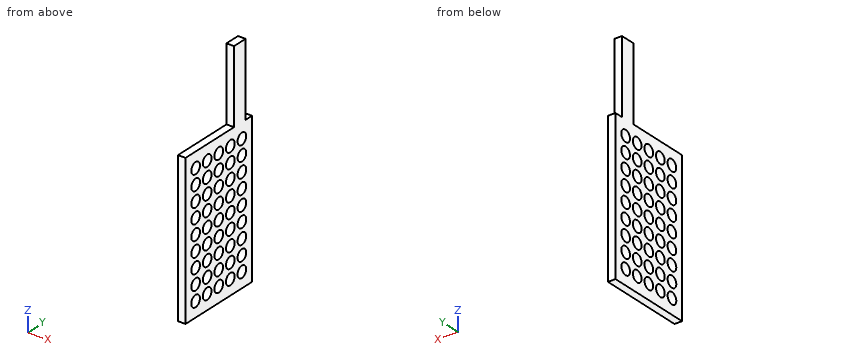
```python
from build123d import *

# Parameters (mm, degrees)
F0_R     = 0.75
F0_W     = 2
F0_H     = 9.755
F1_DEPTH = 1


# Not quite as in the source:
# - a feature names something its author has since deleted; it is built from what else it names


with BuildPart() as f1:
    # F0 (on Right) → F1 (new body)
    with BuildSketch(Plane.YZ):
        Polygon((0, 0.245), (0, 0), (0, -19.7439561955), (11.5, -19.7439561955), (11.5, 0), (11.5, 0.245), (10.384144865, 0.245), (8.384144865, 0.245), (1.75, 0.245), align=None)
        with Locations((1.7424730282, -17.7489561955)):
            Circle(F0_R, mode=Mode.SUBTRACT)
        with Locations((1.7446237513, -15.7489573519)):
            Circle(F0_R, mode=Mode.SUBTRACT)
        with Locations((1.7467744744, -13.7489585083)):
            Circle(F0_R, mode=Mode.SUBTRACT)
        with Locations((3.7424718718, -17.7511069186)):
            Circle(F0_R, mode=Mode.SUBTRACT)
        with Locations((5.7424707154, -17.7532576417)):
            Circle(F0_R, mode=Mode.SUBTRACT)
        with Locations((3.7446225949, -15.751108075)):
            Circle(F0_R, mode=Mode.SUBTRACT)
        with Locations((3.746773318, -13.7511092314)):
            Circle(F0_R, mode=Mode.SUBTRACT)
        with Locations((5.7446214385, -15.7532587981)):
            Circle(F0_R, mode=Mode.SUBTRACT)
        with Locations((5.7467721616, -13.7532599545)):
            Circle(F0_R, mode=Mode.SUBTRACT)
        with Locations((1.7489251975, -11.7489596647)):
            Circle(F0_R, mode=Mode.SUBTRACT)
        with Locations((1.75, -9.75)):
            Circle(F0_R, mode=Mode.SUBTRACT)
        with Locations((1.75, -7.75)):
            Circle(F0_R, mode=Mode.SUBTRACT)
        with Locations((1.75, -5.75)):
            Circle(F0_R, mode=Mode.SUBTRACT)
        with Locations((3.7489243397, -11.7505550493)):
            Circle(F0_R, mode=Mode.SUBTRACT)
        with Locations((3.7499997014, -9.7505553384)):
            Circle(F0_R, mode=Mode.SUBTRACT)
        with Locations((5.7489228847, -11.7532611109)):
            Circle(F0_R, mode=Mode.SUBTRACT)
        with Locations((3.75, -7.75)):
            Circle(F0_R, mode=Mode.SUBTRACT)
        with Locations((3.75, -5.75)):
            Circle(F0_R, mode=Mode.SUBTRACT)
        with Locations((7.742469559, -17.7554083647)):
            Circle(F0_R, mode=Mode.SUBTRACT)
        with Locations((7.7446202821, -15.7554095212)):
            Circle(F0_R, mode=Mode.SUBTRACT)
        with Locations((7.7467710052, -13.7554106776)):
            Circle(F0_R, mode=Mode.SUBTRACT)
        with Locations((9.7424684026, -17.7575590878)):
            Circle(F0_R, mode=Mode.SUBTRACT)
        with Locations((9.7446191257, -15.7575602442)):
            Circle(F0_R, mode=Mode.SUBTRACT)
        with Locations((9.7467698488, -13.7575614006)):
            Circle(F0_R, mode=Mode.SUBTRACT)
        with Locations((5.75, -9.75)):
            Circle(F0_R, mode=Mode.SUBTRACT)
        with Locations((7.7489217283, -11.755411834)):
            Circle(F0_R, mode=Mode.SUBTRACT)
        with Locations((7.75, -9.75)):
            Circle(F0_R, mode=Mode.SUBTRACT)
        with Locations((5.75, -7.75)):
            Circle(F0_R, mode=Mode.SUBTRACT)
        with Locations((5.75, -5.75)):
            Circle(F0_R, mode=Mode.SUBTRACT)
        with Locations((7.75, -7.75)):
            Circle(F0_R, mode=Mode.SUBTRACT)
        with Locations((7.75, -5.75)):
            Circle(F0_R, mode=Mode.SUBTRACT)
        with Locations((9.7489205719, -11.7575625571)):
            Circle(F0_R, mode=Mode.SUBTRACT)
        with Locations((9.75, -9.75)):
            Circle(F0_R, mode=Mode.SUBTRACT)
        with Locations((9.75, -7.75)):
            Circle(F0_R, mode=Mode.SUBTRACT)
        with Locations((9.75, -5.75)):
            Circle(F0_R, mode=Mode.SUBTRACT)
        with Locations((1.75, -3.75)):
            Circle(F0_R, mode=Mode.SUBTRACT)
        with Locations((1.75, -1.75)):
            Circle(F0_R, mode=Mode.SUBTRACT)
        with Locations((3.75, -3.75)):
            Circle(F0_R, mode=Mode.SUBTRACT)
        with Locations((3.75, -1.75)):
            Circle(F0_R, mode=Mode.SUBTRACT)
        with Locations((5.75, -3.75)):
            Circle(F0_R, mode=Mode.SUBTRACT)
        with Locations((5.75, -1.75)):
            Circle(F0_R, mode=Mode.SUBTRACT)
        with Locations((7.75, -3.75)):
            Circle(F0_R, mode=Mode.SUBTRACT)
        with Locations((7.7499570354, -1.7564534015)):
            Circle(F0_R, mode=Mode.SUBTRACT)
        with Locations((9.75, -3.75)):
            Circle(F0_R, mode=Mode.SUBTRACT)
        with Locations((9.75, -1.75)):
            Circle(F0_R, mode=Mode.SUBTRACT)
        with Locations((9.384144865, 5.1225)):
            Rectangle(F0_W, F0_H)
    extrude(amount=F1_DEPTH)


solid = f1.part
```
The listing builds one solid part. Answer for the finished solid, in the listing's coordinates (mm). Give positions to 0.01 mm unless a question says otherwise; leave off trailing zeros. Write each loop counter-clockwise with the first axis right and the second up, starting at its lowest first coordinate (ties: lowest second). Pieces come first, ordered by that corner, then holes. Notation, with made-up numbers: (11.5, 32) -> (26.5, 32) arc R28 cw to (26.5, 69) -> close; hole circle Ø10 at (41, 72.5). An arc over 180 degrees is marked (long way). Write item = value, one per line. Start each with the question number.
1) The part is cut by section B-B, the plane z = 2. Determine the outline of the cut face in (x, y), and give its area (3 significant figures).
2) This flat-tipped pin is pushed along its axis until it touches: pin 1 (2.5 mm diameter, centred on y = 9.74, z = -17.76, fed in from -X). Where does it stop, or does it pass through?
3) Straight lines are drawn through the part: line 1 along Y through (x, z) = (0.6, -2); line 2 along Y through (x, z) = (0.4, 6.5); line 3 along Y through (x, z) = (0.5, -14.25). For each, find the intervals that lie inside material, in ascending order.
4) The part is cut by section A-A, the plane z = -7.75. Determine the outline of the cut face in (x, y), and give its area (3 significant figures).
5) The part is cut by section C-C, the plane y = 3.75. Count the separate pieces of the cut face and the enclosed holes in it, and give its area (3 significant figures).
Solutions:
q1.outline = (0, 8.38) -> (1, 8.38) -> (1, 10.38) -> (0, 10.38) -> close
q1.area = 2.00 mm²
q2.pin_1 = 0
q3.line_1 = 0 to 1.04, 2.46 to 3.04, 4.46 to 5.04, 6.46 to 7.04, 8.46 to 9.04, 10.46 to 11.5
q3.line_2 = 8.38 to 10.38
q3.line_3 = 0 to 1.19, 2.3 to 3.19, 4.31 to 5.18, 6.31 to 7.18, 8.31 to 9.18, 10.31 to 11.5
q4.outline = (0, 0) -> (1, 0) -> (1, 1) -> (0, 1) -> close; (0, 2.5) -> (1, 2.5) -> (1, 3) -> (0, 3) -> close; (0, 4.5) -> (1, 4.5) -> (1, 5) -> (0, 5) -> close; (0, 6.5) -> (1, 6.5) -> (1, 7) -> (0, 7) -> close; (0, 8.5) -> (1, 8.5) -> (1, 9) -> (0, 9) -> close; (0, 10.5) -> (1, 10.5) -> (1, 11.5) -> (0, 11.5) -> close
q4.area = 4.00 mm²
q5.separate_pieces = 10
q5.enclosed_holes = 0
q5.area = 6.49 mm²
